from build123d import *

# Parameters (mm, degrees)
SKETCH_1_R          = 7.5
EXTRUDE_1_DEPTH     = 4
SKETCH_2_R          = 5
EXTRUDE_2_DEPTH     = 13
SKETCH_3_R          = 3.1
EXTRUDE_3_DEPTH     = 2
SKETCH_4_R          = 4
EXTRUDE_4_DEPTH     = 6
SKETCH_6_W          = 2
SKETCH_6_H          = 15.894764062
CUT_EXTRUDE_2_DEPTH = 2


# Read off the part's stored shape, not the designer's step: M8 机械螺纹 螺柱1
with BuildPart() as part:
    # 草图1 → 凸台-拉伸1 (new body)
    with BuildSketch(Plane.XY):
        Circle(SKETCH_1_R)
    extrude(amount=EXTRUDE_1_DEPTH)

    # 草图2 → 凸台-拉伸2 (add)
    with BuildSketch(Plane.XY.offset(4)):
        with Locations(Location((0, 0, 0), (0, 0, 180))):
            Circle(SKETCH_2_R)
    extrude(amount=EXTRUDE_2_DEPTH)

    # 草图3 → 凸台-拉伸3 (add)
    with BuildSketch(Plane.XY.offset(17)):
        Circle(SKETCH_3_R)
    extrude(amount=EXTRUDE_3_DEPTH)

    # 草图4 → 凸台-拉伸4 (add)
    with BuildSketch(Plane.XY.offset(19)):
        Circle(SKETCH_4_R)
    extrude(amount=EXTRUDE_4_DEPTH)

    # M8 机械螺纹 螺柱1 outline → M8 机械螺纹 螺柱1 (revolve, cut)
    with BuildSketch(Plane.XZ):
        Polygon((4, 25), (3.3235, 25), (4, 24.3235), align=None)
    revolve(axis=Axis((0, 0, 0), (0, 0, 1)), mode=Mode.SUBTRACT)

    # 草图6 → 切除-拉伸-薄壁2 (cut)
    with BuildSketch(Plane(origin=(0, 0, 0), x_dir=(-1, 0, 0), z_dir=(0, 0, -1))):
        with Locations((0, 0.006874898)):
            Rectangle(SKETCH_6_W, SKETCH_6_H)
    extrude(amount=-CUT_EXTRUDE_2_DEPTH, mode=Mode.SUBTRACT)


solid = part.part
Input: part model. Units: mm. Frame: model coordinates. A direction names the side the tool comes from. Give positions to 0.01 mm unless a question says otherwise; leave off trailing zeros. Loops run counter-clockwise (first coordinate to the right, second up) from the corner with the lowest first, then second, coordinate; pieces in that order, holes last. Notation, with made-up numbers: (77.25, 87) -> (92.25, 87) arc R19 ccw to (92.25, 101) -> close; hole circle Ø6 at (14.25, 58.5). An arc over 180 degrees is marked (long way). Answer as a JSON object with one key per item and string values. Group by question number.
Item 1: Line query: probe 1 along Z at (x, y) = (0.5, 1.5); probe 2 along Z at (x, y) = (-6, 2); probe 3 along Y at (x, z) = (-3, 7.75). Output: solid intervals per line, ascending.
Item 2: Pull-direction query (Z, two-part tool) for faces 5 (the flat face through (3, 0, 0)), 6 (the cylindrical face through (-1.63, -7.32, 1.97)), 7 (the flat face through (0, 0, 25)), 8 (the flat face through (0.1, 3.3, 17)); classes: released by +Z, released by -Z, zero draft, split by the parting line, or undercut.
Item 3: Reachability of faces 1 (the flat face through (1, 0, 1)), 2 (the flat face through (-4, 0, 0)), 3 (the flat face through (2, -3, 19)), 4 (the cylindrical face through (5, 0, 10)) from +Z, -Z, +X, -X, +Y, -Y: full face, straight path, thin tool, end or side. Return the list, or none.
Item 4: Cut plane B-B, the plane y = 0. Return the cut outline in (x, z), and give its area (3 significant figures).
Item 5: Cut plane C-C, the plane z = 7. Return the cut outline in (x, y).
Item 6: Pin query (flat end, axial travel): P1, Ø2, axis at x = -4, z = 14, coming from the +Y side; P2, Ø2, axis at x = -3, y = -3.5, coming from the +Z side; P3, Ø2, axis at y = 2.5, z = 1, coming from the +X side; P4, Ø2, axis at x = -1, y = 1, coming from the -Z side. Return the tip coordinate at first contact, or that it passes through.
Item 7: Cut plane A-A, the plane x = 0. Return the cut outline in (y, z).
Item 8: Cut plane D-D, the plane y = 6. Return the cut outline in (x, z), and give its area (3 significant figures).
Checks:
{
 "1": {"probe 1": "z = 2 to 25", "probe 2": "z = 0 to 4", "probe 3": "y = -4 to 4"},
 "2": {"face 5": "released by -Z", "face 6": "zero draft", "face 7": "released by +Z", "face 8": "undercut"},
 "3": {"face 1": "-Z, +Y, -Y", "face 2": "-Z, +X, -X, +Y, -Y", "face 3": "none", "face 4": "+Z"},
 "4": {"outline": "(-7.5, 0) -> (-1, 0) -> (-1, 2) -> (1, 2) -> (1, 0) -> (7.5, 0) -> (7.5, 4) -> (5, 4) -> (5, 17) -> (3.1, 17) -> (3.1, 19) -> (4, 19) -> (4, 24.32) -> (3.32, 25) -> (-3.32, 25) -> (-4, 24.32) -> (-4, 19) -> (-3.1, 19) -> (-3.1, 17) -> (-5, 17) -> (-5, 4) -> (-7.5, 4) -> close", "area": "246 mm²"},
 "5": {"outline": "circle Ø10 at (0, 0)"},
 "6": {"P1": "stops at y = 4", "P2": "stops at z = 24.71", "P3": "stops at x = 7.35", "P4": "stops at z = 0"},
 "7": {"outline": "(-7.5, 2) -> (7.5, 2) -> (7.5, 4) -> (5, 4) -> (5, 17) -> (3.1, 17) -> (3.1, 19) -> (4, 19) -> (4, 24.32) -> (3.32, 25) -> (-3.32, 25) -> (-4, 24.32) -> (-4, 19) -> (-3.1, 19) -> (-3.1, 17) -> (-5, 17) -> (-5, 4) -> (-7.5, 4) -> close"},
 "8": {"outline": "(-4.5, 0) -> (-1, 0) -> (-1, 2) -> (1, 2) -> (1, 0) -> (4.5, 0) -> (4.5, 4) -> (-4.5, 4) -> close", "area": "32.0 mm²"}
}
